Verification items for the finished model (mm, model axes). Coordinates: 2 decimals unless noted, no trailing zeros. Write item = value, one per line. Start each with the question number.
(1) Section check A-A (y = 0.95). State how many separate pieces and enclosed holes the cut face has, plus the area to 3 significant figures.
(2) Gauge pin test, flat ends, axial feed: pin 1 Ø2.5 at (x, y) = (45, 2.5) entering from +Z; pin 2 Ø1.4 at (y, z) = (1.5, -40.5) entering from +X; pin 3 Ø5 at (x, z) = (-43.66, 27.05) entering from +Y. Record the tip position at first contact, or that the pin passes through.
(3) Material ranges on probe 1 along X at (y, z) = (3, -35); probe 2 along X at (y, z) = (4.2, -25.5); probe 3 along Z at (x, y) = (42.5, 3.7), recorded low to high. Write a range as [from, to].
```python
from build123d import *

# Parameters (mm, degrees)
SKETCH1_R           = 1.524
BOSS_EXTRUDE1_DEPTH = 4.7625
CHAMFER1_SIZE       = 1.490392112
CHAMFER1_SIZE_2     = 1.7145


with BuildPart() as part:
    # Sketch1 → Boss-Extrude1 (new body)
    with BuildSketch(Plane(origin=(0, 0, 0), x_dir=(1, 0, 0), z_dir=(0, 1, 0))):
        Polygon((-41.1226, 44.45), (41.1226, 44.45), (41.1226, 34.7726), (46.0375, 34.7726), (46.0375, -34.7726), (41.1226, -34.7726), (41.1226, -46.0375), (-41.1226, -46.0375), (-41.1226, -34.7726), (-46.0375, -34.7726), (-46.0375, 34.7726), (-41.1226, 34.7726), align=None)
        with Locations(Location((43.65625, 27.051, 0), (0, 0, 90))):
            Circle(SKETCH1_R, mode=Mode.SUBTRACT)
        with Locations(Location((43.65625, -27.051, 0), (0, 0, 90))):
            Circle(SKETCH1_R, mode=Mode.SUBTRACT)
        with Locations(Location((-43.65625, -27.051, 0), (0, 0, 90))):
            Circle(SKETCH1_R, mode=Mode.SUBTRACT)
        with Locations(Location((-43.65625, 27.051, 0), (0, 0, 90))):
            Circle(SKETCH1_R, mode=Mode.SUBTRACT)
    extrude(amount=BOSS_EXTRUDE1_DEPTH)

    # Chamfer1
    # the kernel refuses this chamfer: 1.7145, 1.490392112 mm, written as the material it takes off along each edge
    with BuildSketch(Plane(origin=(43.65625, 4.7625, -27.051), x_dir=(0, 0, -1), z_dir=(1, 0, 0))) as chamfer1_piece_1:
        Polygon((1.524, -CHAMFER1_SIZE), (1.524 + CHAMFER1_SIZE_2, 0), (1.524, 0), align=None)
    revolve(axis=Axis((43.65625, 4.7625, -27.051), (0, 1, 0)), mode=Mode.SUBTRACT)
    with BuildSketch(Plane(origin=(43.65625, 4.7625, 27.051), x_dir=(0, 0, -1), z_dir=(1, 0, 0))) as chamfer1_piece_2:
        Polygon((1.524, -CHAMFER1_SIZE), (1.524 + CHAMFER1_SIZE_2, 0), (1.524, 0), align=None)
    revolve(axis=Axis((43.65625, 4.7625, 27.051), (0, 1, 0)), mode=Mode.SUBTRACT)
    with BuildSketch(Plane(origin=(-43.65625, 4.7625, 27.051), x_dir=(0, 0, -1), z_dir=(1, 0, 0))) as chamfer1_piece_3:
        Polygon((1.524, -CHAMFER1_SIZE), (1.524 + CHAMFER1_SIZE_2, 0), (1.524, 0), align=None)
    revolve(axis=Axis((-43.65625, 4.7625, 27.051), (0, 1, 0)), mode=Mode.SUBTRACT)
    with BuildSketch(Plane(origin=(-43.65625, 4.7625, -27.051), x_dir=(0, 0, -1), z_dir=(1, 0, 0))) as chamfer1_piece_4:
        Polygon((1.524, -CHAMFER1_SIZE), (1.524 + CHAMFER1_SIZE_2, 0), (1.524, 0), align=None)
    revolve(axis=Axis((-43.65625, 4.7625, -27.051), (0, 1, 0)), mode=Mode.SUBTRACT)


solid = part.part
```
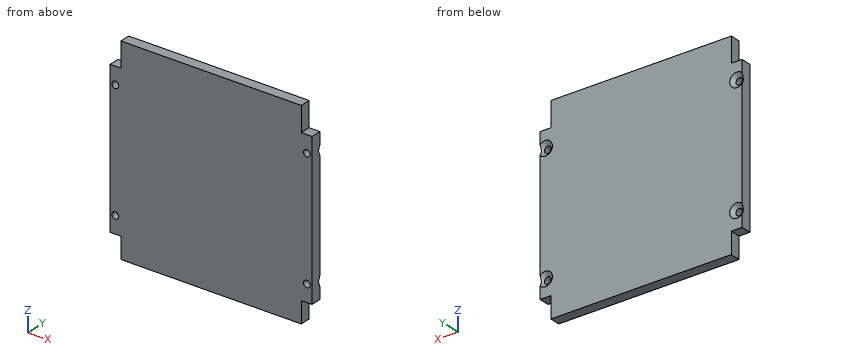
Response:
q1.separate_pieces = 1
q1.enclosed_holes = 4
q1.area = 8,100 mm2
q2.pin_1 = 34.77
q2.pin_2 = 41.12
q2.pin_3 = 4.12
q3.probe_1 = [-41.12, 41.12]
q3.probe_2 = [-46.04, -45.73], [-41.58, 41.58], [45.73, 46.04]
q3.probe_3 = [-34.77, -28.7], [-25.4, 25.4], [28.7, 34.77]
